from build123d import *

# Parameters (mm, degrees)
F1_DEPTH = 15
F0_R     = 1
F2_DEPTH = 1.5


with BuildPart() as f1:
    # F0 (on Top) → F1 (new body)
    with BuildSketch(Plane.XY):
        with BuildLine():
            Line((-13.388073, -19.039594), (-13.388073, -2.839899))
            ThreePointArc((-13.388073, -2.839899), (-29.757069, 2.654483), (-46.126065, -2.839899))
            Line((-46.126065, -2.839899), (-46.126065, -19.039594))
            ThreePointArc((-46.126065, -19.039594), (-29.757069, -24.533976), (-13.388073, -19.039594))
        make_face()
        with BuildLine():
            ThreePointArc((-45.16989, -3.320836), (-29.757069, 1.698308), (-14.344248, -3.320836))
            Line((-14.344248, -3.320836), (-14.344248, -18.558657))
            ThreePointArc((-14.344248, -18.558657), (-29.757069, -23.577801), (-45.16989, -18.558657))
            Line((-45.16989, -18.558657), (-45.16989, -3.320836))
        make_face(mode=Mode.SUBTRACT)
    extrude(amount=F1_DEPTH)

    # F0 (on Top) → F2 (join)
    with BuildSketch(Plane.XY):
        with BuildLine():
            Line((-14.344248, -18.558657), (-14.344248, -3.320836))
            ThreePointArc((-14.344248, -3.320836), (-29.757069, 1.698308), (-45.16989, -3.320836))
            Line((-45.16989, -3.320836), (-45.16989, -18.558657))
            ThreePointArc((-45.16989, -18.558657), (-29.757069, -23.577801), (-14.344248, -18.558657))
        make_face()
        with Locations((-38.523632, -19.683723)):
            Circle(F0_R, mode=Mode.SUBTRACT)
        with Locations((-35.023632, -19.683723)):
            Circle(F0_R, mode=Mode.SUBTRACT)
        with Locations((-31.523632, -19.683723)):
            Circle(F0_R, mode=Mode.SUBTRACT)
        with Locations((-42.023632, -16.183723)):
            Circle(F0_R, mode=Mode.SUBTRACT)
        with Locations((-38.523632, -16.183723)):
            Circle(F0_R, mode=Mode.SUBTRACT)
        with Locations((-42.023632, -12.683723)):
            Circle(F0_R, mode=Mode.SUBTRACT)
        with Locations((-38.523632, -12.683723)):
            Circle(F0_R, mode=Mode.SUBTRACT)
        with Locations((-35.023632, -16.183723)):
            Circle(F0_R, mode=Mode.SUBTRACT)
        with Locations((-31.523632, -16.183723)):
            Circle(F0_R, mode=Mode.SUBTRACT)
        with Locations((-35.023632, -12.683723)):
            Circle(F0_R, mode=Mode.SUBTRACT)
        with Locations((-31.523632, -12.683723)):
            Circle(F0_R, mode=Mode.SUBTRACT)
        with Locations((-28.023632, -19.683723)):
            Circle(F0_R, mode=Mode.SUBTRACT)
        with Locations((-24.523632, -19.683723)):
            Circle(F0_R, mode=Mode.SUBTRACT)
        with Locations((-21.023632, -19.683723)):
            Circle(F0_R, mode=Mode.SUBTRACT)
        with Locations((-28.023632, -16.183723)):
            Circle(F0_R, mode=Mode.SUBTRACT)
        with Locations((-24.523632, -16.183723)):
            Circle(F0_R, mode=Mode.SUBTRACT)
        with Locations((-28.023632, -12.683723)):
            Circle(F0_R, mode=Mode.SUBTRACT)
        with Locations((-24.523632, -12.683723)):
            Circle(F0_R, mode=Mode.SUBTRACT)
        with Locations((-21.023632, -16.183723)):
            Circle(F0_R, mode=Mode.SUBTRACT)
        with Locations((-17.523632, -16.183723)):
            Circle(F0_R, mode=Mode.SUBTRACT)
        with Locations((-21.023632, -12.683723)):
            Circle(F0_R, mode=Mode.SUBTRACT)
        with Locations((-17.523632, -12.683723)):
            Circle(F0_R, mode=Mode.SUBTRACT)
        with Locations((-42.023632, -9.183723)):
            Circle(F0_R, mode=Mode.SUBTRACT)
        with Locations((-38.523632, -9.183723)):
            Circle(F0_R, mode=Mode.SUBTRACT)
        with Locations((-42.023632, -5.683723)):
            Circle(F0_R, mode=Mode.SUBTRACT)
        with Locations((-38.523632, -5.683723)):
            Circle(F0_R, mode=Mode.SUBTRACT)
        with Locations((-35.023632, -9.183723)):
            Circle(F0_R, mode=Mode.SUBTRACT)
        with Locations((-31.523632, -9.183723)):
            Circle(F0_R, mode=Mode.SUBTRACT)
        with Locations((-35.023632, -5.683723)):
            Circle(F0_R, mode=Mode.SUBTRACT)
        with Locations((-31.523632, -5.683723)):
            Circle(F0_R, mode=Mode.SUBTRACT)
        with Locations((-38.523632, -2.183723)):
            Circle(F0_R, mode=Mode.SUBTRACT)
        with Locations((-35.023632, -2.183723)):
            Circle(F0_R, mode=Mode.SUBTRACT)
        with Locations((-31.523632, -2.183723)):
            Circle(F0_R, mode=Mode.SUBTRACT)
        with Locations((-28.023632, -9.183723)):
            Circle(F0_R, mode=Mode.SUBTRACT)
        with Locations((-24.523632, -9.183723)):
            Circle(F0_R, mode=Mode.SUBTRACT)
        with Locations((-28.023632, -5.683723)):
            Circle(F0_R, mode=Mode.SUBTRACT)
        with Locations((-24.523632, -5.683723)):
            Circle(F0_R, mode=Mode.SUBTRACT)
        with Locations((-21.023632, -9.183723)):
            Circle(F0_R, mode=Mode.SUBTRACT)
        with Locations((-17.523632, -9.183723)):
            Circle(F0_R, mode=Mode.SUBTRACT)
        with Locations((-21.023632, -5.683723)):
            Circle(F0_R, mode=Mode.SUBTRACT)
        with Locations((-17.523632, -5.683723)):
            Circle(F0_R, mode=Mode.SUBTRACT)
        with Locations((-28.023632, -2.183723)):
            Circle(F0_R, mode=Mode.SUBTRACT)
        with Locations((-24.523632, -2.183723)):
            Circle(F0_R, mode=Mode.SUBTRACT)
        with Locations((-21.023632, -2.183723)):
            Circle(F0_R, mode=Mode.SUBTRACT)
    extrude(amount=F2_DEPTH)


solid = f1.part
Input: part model. Units: mm. Frame: model coordinates. A direction names the side the tool comes from. Give positions to 0.01 mm unless a question says otherwise; leave off trailing zeros. Write each loop counter-clockwise with the first axis right and the second up, starting at its lowest first coordinate (ties: lowest second). Pieces come first, ordered by that corner, then holes. Notation, with made-up numbers: M 54.5,-39 L 97.5,-39 A22 ccw 97.5,-2 Z; hole C 5.25,-3 d11. An arc over 180 degrees is marked long. Write item = value, one per line. Start each with the question number.
1) Draft query along Y for faces 3 (the flat face through (-30, -11, 0)), 4 (the cylindrical face through (-29.511, 2.653, 7.395)), 5 (the flat face through (-45.17, -11, 8)). Return one class per face: +Y half, -Y half, draft (parallel to the pull), parting line (faces both ways), or undercut.
2) Material intervals for line 1 along X through (y, z) = (-17, 2.25); line 2 along Z through (x, y) = (-37, -0.5); line 3 along X through (y, z) = (-2.5, 6.25), sorted ascending. Write a range as [from, to].
3) Cut plane B-B on x = -32. Count the separate pieces of the cut face and the enclosed holes in it, then the cut area to 3 significant figures.
4) First-contact query: pin 1 Ø2.5 at (x, y) = (-21.02, -9.18) entering from +Z; pin 2 Ø8 at (x, z) = (-24.5, 9.5) entering from +Y; pin 3 Ø1.8 at (x, y) = (-35.02, -9.18) entering from +Z; pin 4 Ø2 at (x, z) = (-26, 3) entering from +Y. Flat tips, straight axial feed; report the tip coordinate or a pass-through.
5) Cut plane D-D on x = -44. Return the cut outline in (y, z), then the cut area to 3 significant figures.
6) Reachability of faces 1 (the cylindrical face through (-27.1, -20.07, 0.74)), 2 (the cylindrical face through (-29.526, -23.577, 8.156)) from +Z, -Z, +X, -X, +Y, -Y: full face, straight path, thin tool, end or side. Return the list, or none.
7) Cut plane A-A on z = 13. Return the cut outline in (x, y), then the cut area to 3 significant figures.
Solved:
q1.face_3 = draft
q1.face_4 = +Y half
q1.face_5 = undercut
q2.line_1 = [-46.13, -45.17], [-14.34, -13.39]
q2.line_2 = [0, 1.5]
q2.line_3 = [-45.67, -43.98], [-15.54, -13.85]
q3.separate_pieces = 7
q3.enclosed_holes = 0
q3.area = 50.6 mm2
q4.pin_1 = 1.5
q4.pin_2 = 2.63
q4.pin_3 = through
q4.pin_4 = 2.51
q5.outline = M -20.49,0 L -1.38,0 L -1.38,15 L -2.52,15 L -2.52,1.5 L -19.36,1.5 L -19.36,15 L -20.49,15 Z
q5.area = 59.2 mm2
q6.face_1 = +Z, -Z
q6.face_2 = +Z
q7.outline = M -46.13,-19.04 A27.13 ccw -13.39,-19.04 L -13.39,-2.84 A27.13 ccw -46.13,-2.84 Z; hole M -45.17,-18.56 A26.17 ccw -14.34,-18.56 L -14.34,-3.32 A26.17 ccw -45.17,-3.32 Z
q7.area = 95.2 mm2
